Work out the finished part from the listing and answer in its coordinate system (mm). A direction names the side the tool comes from. Coordinates: 2 decimals unless noted, no trailing zeros. Loops run counter-clockwise (first coordinate to the right, second up) from the corner with the lowest first, then second, coordinate; pieces in that order, holes last.
```python
from build123d import *

# Parameters (mm, degrees)
SKETCH1_W                      = 41
SKETCH1_H                      = 33.02
SKETCH1_R                      = 3.175
BOSS_EXTRUDE1_DEPTH            = 12
SKETCH2_W                      = 41
SKETCH2_H                      = 7.62
BOSS_EXTRUDE2_DEPTH            = 53
CUT_EXTRUDE1_REACH             = 72.127
SKETCH4_R                      = 3.175
CUT_EXTRUDE1_DIRECTION_2_REACH = 72.127
CUT_EXTRUDE3_REACH             = 72.127
CUT_EXTRUDE3_DIRECTION_2_REACH = 72.127
FILLET1_R                      = 10
CUT_EXTRUDE4_DEPTH             = 5.08


with BuildPart() as part:
    # Sketch1 → Boss-Extrude1 (new body)
    with BuildSketch(Plane.XY):
        Rectangle(SKETCH1_W, SKETCH1_H)
        with Locations((12.5, 0)):
            Circle(SKETCH1_R, mode=Mode.SUBTRACT)
        with Locations((-12.5, 0)):
            Circle(SKETCH1_R, mode=Mode.SUBTRACT)
    extrude(amount=BOSS_EXTRUDE1_DEPTH)

    # Sketch2 → Boss-Extrude2 (add)
    with BuildSketch(Plane.XY.offset(12)):
        with Locations((0, 12.7)):
            Rectangle(SKETCH2_W, SKETCH2_H)
        with Locations((0, -12.7)):
            Rectangle(SKETCH2_W, SKETCH2_H)
    extrude(amount=BOSS_EXTRUDE2_DEPTH)

    # Cut-Extrude1: up to this face of the body (flat: up to its plane)
    cut_extrude1_end = Plane(part.part.faces().sort_by_distance((0, -16.51, 32.5))[0])
    # Sketch4 → Cut-Extrude1 (cut, up to the picked face)
    with BuildSketch(Plane(origin=(0, 0, 0), x_dir=(1, 0, 0), z_dir=(0, 1, 0)), mode=Mode.PRIVATE) as cut_extrude1_sk1:
        with Locations(Location((0, -35.5, 0), (0, 0, 270))):
            Circle(SKETCH4_R)
    cut_extrude1_tool1 = split(extrude(cut_extrude1_sk1.sketch, amount=-CUT_EXTRUDE1_REACH, mode=Mode.PRIVATE), bisect_by=cut_extrude1_end, keep=Keep.BOTH, mode=Mode.PRIVATE)
    add(cut_extrude1_tool1.solids().sort_by(Axis((0, 0, 35.5), (0, -1, 0)))[0], mode=Mode.SUBTRACT)

    # Cut-Extrude1 direction 2: up to this face of the body (flat: up to its plane)
    cut_extrude1_direction_2_end = Plane(part.part.faces().sort_by_distance((0, 16.51, 32.5))[0])
    # Sketch4 → Cut-Extrude1 direction 2 (cut, up to the picked face)
    with BuildSketch(Plane(origin=(0, 0, 0), x_dir=(1, 0, 0), z_dir=(0, 1, 0)), mode=Mode.PRIVATE) as cut_extrude1_direction_2_sk1:
        with Locations(Location((0, -35.5, 0), (0, 0, 270))):
            Circle(SKETCH4_R)
    cut_extrude1_direction_2_tool1 = split(extrude(cut_extrude1_direction_2_sk1.sketch, amount=CUT_EXTRUDE1_DIRECTION_2_REACH, mode=Mode.PRIVATE), bisect_by=cut_extrude1_direction_2_end, keep=Keep.BOTH, mode=Mode.PRIVATE)
    add(cut_extrude1_direction_2_tool1.solids().sort_by(Axis((0, 0, 35.5), (0, 1, 0)))[0], mode=Mode.SUBTRACT)

    # Cut-Extrude3: up to this face of the body (flat: up to its plane)
    cut_extrude3_end = Plane(part.part.faces().sort_by_distance((-19.731494958, -16.51, 32.5))[0])
    # Sketch6 → Cut-Extrude3 (cut, up to the picked face)
    with BuildSketch(Plane(origin=(0, 0, 0), x_dir=(1, 0, 0), z_dir=(0, 1, 0)), mode=Mode.PRIVATE) as cut_extrude3_sk1:
        with BuildLine():
            Line((-8, -35.5), (-8, -20))
            ThreePointArc((-8, -20), (-10.343145751, -14.343145751), (-16, -12))
            Line((-16, -12), (-20.5, -12))
            Line((-20.5, -12), (-20.5, -65))
            Line((-20.5, -65), (20.5, -65))
            Line((20.5, -65), (20.5, -12))
            Line((20.5, -12), (16, -12))
            ThreePointArc((16, -12), (10.343145751, -14.343145751), (8, -20))
            Line((8, -20), (8, -35.5))
            ThreePointArc((8, -35.5), (0, -43.5), (-8, -35.5))
        make_face()
    cut_extrude3_tool1 = split(extrude(cut_extrude3_sk1.sketch, amount=-CUT_EXTRUDE3_REACH, mode=Mode.PRIVATE), bisect_by=cut_extrude3_end, keep=Keep.BOTH, mode=Mode.PRIVATE)
    add(cut_extrude3_tool1.solids().sort_by(Axis((-8.670075, 0, 27.75), (0, -1, 0)))[0], mode=Mode.SUBTRACT)

    # Cut-Extrude3 direction 2: up to this face of the body (flat: up to its plane)
    cut_extrude3_direction_2_end = Plane(part.part.faces().sort_by_distance((19.731494958, 16.51, 32.5))[0])
    # Sketch6 → Cut-Extrude3 direction 2 (cut, up to the picked face)
    with BuildSketch(Plane(origin=(0, 0, 0), x_dir=(1, 0, 0), z_dir=(0, 1, 0)), mode=Mode.PRIVATE) as cut_extrude3_direction_2_sk1:
        with BuildLine():
            Line((-8, -35.5), (-8, -20))
            ThreePointArc((-8, -20), (-10.343145751, -14.343145751), (-16, -12))
            Line((-16, -12), (-20.5, -12))
            Line((-20.5, -12), (-20.5, -65))
            Line((-20.5, -65), (20.5, -65))
            Line((20.5, -65), (20.5, -12))
            Line((20.5, -12), (16, -12))
            ThreePointArc((16, -12), (10.343145751, -14.343145751), (8, -20))
            Line((8, -20), (8, -35.5))
            ThreePointArc((8, -35.5), (0, -43.5), (-8, -35.5))
        make_face()
    cut_extrude3_direction_2_tool1 = split(extrude(cut_extrude3_direction_2_sk1.sketch, amount=CUT_EXTRUDE3_DIRECTION_2_REACH, mode=Mode.PRIVATE), bisect_by=cut_extrude3_direction_2_end, keep=Keep.BOTH, mode=Mode.PRIVATE)
    add(cut_extrude3_direction_2_tool1.solids().sort_by(Axis((-8.670075, 0, 27.75), (0, 1, 0)))[0], mode=Mode.SUBTRACT)

    # Fillet1
    fillet1_edges = [part.edges().sort_by_distance(p)[0] for p in [
        (-20.5, -16.51, 6),
        (-20.5, 16.51, 6),
        (20.5, -16.51, 6),
        (20.5, 16.51, 6),
    ]]
    fillet(fillet1_edges, radius=FILLET1_R)

    # Sketch7 → Cut-Extrude4 (cut)
    with BuildSketch(Plane(origin=(0, 0, 0), x_dir=(-1, 0, 0), z_dir=(0, 0, -1))):
        with BuildLine():
            Line((-10.5, -16.51), (10.5, -16.51))
            ThreePointArc((10.5, -16.51), (17.571067812, -13.581067812), (20.5, -6.51))
            Line((20.5, -6.51), (20.5, 6.51))
            ThreePointArc((20.5, 6.51), (17.571067812, 13.581067812), (10.5, 16.51))
            Line((10.5, 16.51), (-10.5, 16.51))
            ThreePointArc((-10.5, 16.51), (-17.571067812, 13.581067812), (-20.5, 6.51))
            Line((-20.5, 6.51), (-20.5, -6.51))
            ThreePointArc((-20.5, -6.51), (-17.571067812, -13.581067812), (-10.5, -16.51))
        make_face()
    extrude(amount=-CUT_EXTRUDE4_DEPTH, mode=Mode.SUBTRACT)


solid = part.part
```
1. For faces 4 (the flat face through (-8, -13, 28)), 5 (the cylindrical face through (10.406, 12.647, 14.281)), determine the directions among +Z, -Z, +X, -X, +Y, -Y from which every point of the face is accessible in a straight line to the end or side of a thin tool.
2. Straight lines are drawn through the part: probe 1 along X at (y, z) = (0, 7.5) (3 decimals); probe 2 along Y at (x, z) = (-3, 14.5); probe 3 along X at (y, z) = (12.5, 35.5) (3 decimals). For each, find the intervals that lie inside material, in ascending order.
3. A cutting plane is placed at C-C, the plane z = 39.5. Give the vertices of the cut face in (x, y), then the cut area to 3 significant figures.
4. A cutting plane is placed at B-B, the plane x = 0. Give the vertices of the cut face in (y, z) (3 decimals), then the cut area to 3 significant figures.
5. Determine the mould class of faces 1 (the flat face through (0, 8.89, 28)), 2 (the cylindrical face through (17.65, 13.5, 8.56)), 3 (the cylindrical face through (17.65, -13.5, 8.56)) for opening direction Y: released by +Y, released by -Y, zero draft, split by the parting line, or undercut.
6. A cutting plane is placed at D-D, the plane y = 13. Give the vertices of the cut face in (x, z) (3 decimals).
7. Each of these flat-tipped pins is pushed along its axis until it touches: P1, Ø7.5, axis at x = 12.5, y = 0, coming from the -Z side; P2, Ø8.5, axis at y = 11.5, z = 27, coming from the -X side; P3, Ø1, axis at x = -3, y = 7.5, coming from the +Z side; P4, Ø6, axis at y = 11, z = 30.5, coming from the +X side. Where does it stop, or does it pass through?
8. A cutting plane is placed at A-A, the plane y = 0. Give the vertices of the cut face in (x, z) (3 decimals).
Answers below:
1. face 4: +Z, -X, +Y, -Y
1. face 5: +Z, +X, +Y, -Y
2. probe 1: x = -20.5 to -15.675, -9.325 to 9.325, 15.675 to 20.5
2. probe 2: y = -16.51 to -8.89, 8.89 to 16.51
2. probe 3: x = -8 to -3.175, 3.175 to 8
3. outline: (-6.93, -16.51) - (6.93, -16.51) - (6.93, -8.89) - (-6.93, -8.89) - close; (-6.93, 8.89) - (6.93, 8.89) - (6.93, 16.51) - (-6.93, 16.51) - close
3. area: 211 mm2
4. outline: (-16.51, 5.08) - (16.51, 5.08) - (16.51, 32.325) - (8.89, 32.325) - (8.89, 12) - (-8.89, 12) - (-8.89, 32.325) - (-16.51, 32.325) - close; (-16.51, 38.675) - (-8.89, 38.675) - (-8.89, 43.5) - (-16.51, 43.5) - close; (8.89, 38.675) - (16.51, 38.675) - (16.51, 43.5) - (8.89, 43.5) - close
4. area: 612 mm2
5. face 1: undercut
5. face 2: released by +Y
5. face 3: released by -Y
6. outline: (-18.108, 5.08) - (18.108, 5.08) - (18.108, 12) - (16, 12) arc R8 cw to (8, 20) - (8, 35.5) arc R8 ccw to (-8, 35.5) - (-8, 20) arc R8 cw to (-16, 12) - (-18.108, 12) - close; hole circle Ø6.35 at (0, 35.5)
7. P1: stops at z = 5.08
7. P2: stops at x = -8
7. P3: stops at z = 12
7. P4: stops at x = 8
8. outline: (-20.5, 5.08) - (-15.675, 5.08) - (-15.675, 12) - (-20.5, 12) - close; (-9.325, 5.08) - (9.325, 5.08) - (9.325, 12) - (-9.325, 12) - close; (15.675, 5.08) - (20.5, 5.08) - (20.5, 12) - (15.675, 12) - close
